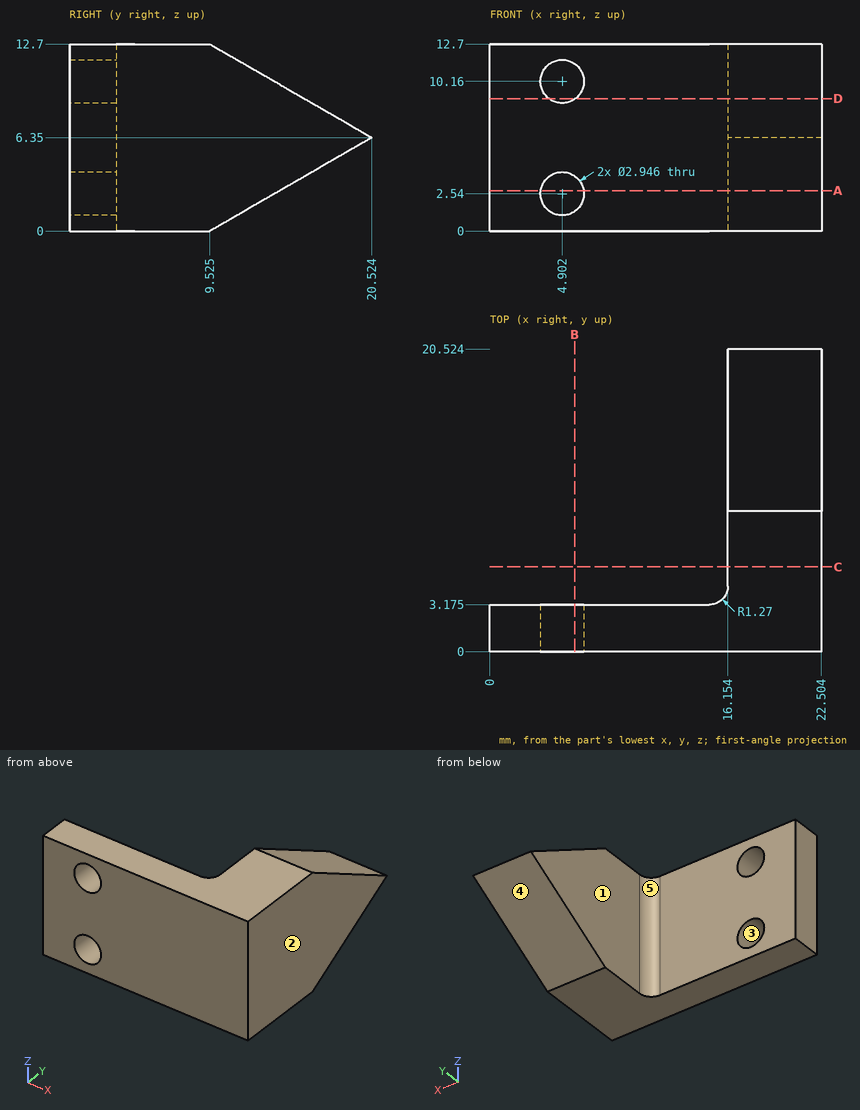
Drawing for the job (mm, zero at the part's lowest x, y, z). A direction names the side the tool comes from. Round coordinates to 2 decimals unless told otherwise and drop trailing zeros. Loops run counter-clockwise (first coordinate to the right, second up) from the corner with the lowest first, then second, coordinate; pieces in that order, holes last. Notation, with made-up numbers: (24, 25.5) - (28, 25.5) arc R13 ccw to (28, 47.5) - close; hole circle Ø10 at (-14.5, 80.25). An arc over 180 degrees is marked (long way). Return JSON: item names as keys, results as strings. Group by question number.
Q1. Band-saw the part on C-C on y = 5.75. Give the cut face in (x, z) (1 decimal).
Q2. Band-saw the part on B-B on x = 5.75. Give the cut face in (y, z) (1 decimal).
Q3. Drill centre lines: line 1 along X through (y, z) = (2.15, 10.16) (1 decimal); line 2 along Y through (x, z) = (10.5, 11.5) (1 decimal); line 3 along X through (y, z) = (8, 10) (1 decimal). Where is each one in solid material? Low to high. Write a range as [from, to].
Q4. Two-plate mould, pull along Z, no slides. Class the marked faces 3, 4 and 5: +Z half, -Z half, draft (parallel to the pull), parting line (faces both ways), or undercut.
Q5. Band-saw the part on A-A on z = 2.75. Give the cut face in (x, y) (1 decimal), plus the area to 3 significant figures.
Q6. Flat gauge pins, fed straight in: pin 1 Ø4 at (x, z) = (4.9, 10.16) entering from +Y (3 decimals); pin 2 Ø6.5 at (y, z) = (9.5, 7.5) entering from -X; pin 3 Ø2 at (x, y) = (14, 6) entering from -Z. Where does each tip first touch, or does it go through?
Q7. Band-saw the part on D-D on z = 9. Give the cut face in (x, y) (1 decimal), plus the area to 3 significant figures.
Q8. Tool access for the marked faces 1 and 2: list every direction of +Z, -Z, +X, -X, +Y, -Y with a clear straight run to the whole face (end or side of a thin tool).
Solutions:
{
 "1": {"outline": "(16.2, 0) - (22.5, 0) - (22.5, 12.7) - (16.2, 12.7) - close"},
 "2": {"outline": "(0, 0) - (3.2, 0) - (3.2, 1.3) - (0, 1.3) - close; (0, 3.7) - (3.2, 3.7) - (3.2, 9) - (0, 9) - close; (0, 11.4) - (3.2, 11.4) - (3.2, 12.7) - (0, 12.7) - close"},
 "3": {"line 1": "x = [0, 3.4], [6.4, 22.5]", "line 2": "y = [0, 3.2]", "line 3": "x = [16.2, 22.5]"},
 "4": {"face 3": "undercut", "face 4": "-Z half", "face 5": "draft"},
 "5": {"outline": "(0, 0) - (3.4, 0) - (3.4, 3.2) - (0, 3.2) - close; (6.4, 0) - (22.5, 0) - (22.5, 14.3) - (16.2, 14.3) - (16.2, 4.4) arc R1.3 cw to (14.9, 3.2) - (6.4, 3.2) - close", "area": "133 mm^2"},
 "6": {"pin 1": "stops at y = 3.175", "pin 2": "stops at x = 16.15", "pin 3": "passes through"},
 "7": {"outline": "(0, 0) - (4, 0) - (4, 3.2) - (0, 3.2) - close; (5.8, 0) - (22.5, 0) - (22.5, 15.9) - (16.2, 15.9) - (16.2, 4.4) arc R1.3 cw to (14.9, 3.2) - (5.8, 3.2) - close", "area": "147 mm^2"},
 "8": {"face 1": "+Z, -Z, -X, +Y", "face 2": "+Z, -Z, +X, +Y, -Y"}
}
